```python
from build123d import *

# Parameters (mm, degrees)
F1_DEPTH  = 12.7
F2_R      = 5.08
F3_SIZE   = 6.34999
F7_DEPTH  = 25.4
F9_DEPTH  = 25.4
F6_R      = 3.175
F10_DEPTH = 25.4


# Not quite as in the source:
# - a fillet or chamfer is up to 0.001 mm smaller than in the source, because OpenCascade refuses the exact size


with BuildPart() as f1:
    # F0 (on Top) → F1 (new body)
    with BuildSketch(Plane.XY):
        with BuildLine():
            ThreePointArc((-85.1017062912, 39.9863691127), (36.5051433715, 149.8230416662), (158.1119930343, 39.9863691127))
            Line((158.1119930343, 39.9863691127), (175.5953490648, 40.6241259528))
            ThreePointArc((175.5953490648, 40.6241259528), (36.5051433715, 167.2855416662), (-102.5850623217, 40.6241259528))
            Line((-102.5850623217, 40.6241259528), (-85.1017062912, 39.9863691127))
        make_face()
    extrude(amount=F1_DEPTH)

    # F2
    f2_edges = [f1.edges().sort_by_distance(p)[0] for p in [
        (36.505143, 167.285542, 12.7),
        (36.505143, 167.285542, 0),
    ]]
    fillet(f2_edges, radius=F2_R)

    # F3 (size 6.35 in the source; OpenCascade refuses exactly that, so slightly less here)
    f3_edges = [f1.edges().sort_by_distance(p)[0] for p in [
        (36.505143, 149.823042, 12.7),
        (36.505143, 149.823042, 0),
    ]]
    chamfer(f3_edges, length=F3_SIZE)


with BuildPart() as f4_1:
    # F4: instance of F1
    add(f1.part.mirror(Plane.XY))


with BuildPart() as f1_1:
    add(f1.part)

    # F6 (on face) → F7 (cut)
    with BuildSketch(Plane.XY.offset(12.7)):
        with BuildLine():
            ThreePointArc((163.0583931619, 73.4856437086), (162.4024850501, 75.2552779595), (161.7218329639, 77.0155431585))
            ThreePointArc((161.7218329639, 77.0155431585), (161.8086296648, 75.0304207129), (163.0583931619, 73.4856437086))
        make_face()
    extrude(amount=-F7_DEPTH, mode=Mode.SUBTRACT)

    # F8 (on face) → F9 (cut)
    with BuildSketch(Plane.XY.offset(12.7)):
        with BuildLine():
            ThreePointArc((64.4226124591, 159.2789709622), (62.573664155, 159.6574032574), (60.7195923208, 160.0098780326))
            ThreePointArc((60.7195923208, 160.0098780326), (62.4506994343, 159.0344227782), (64.4226124591, 159.2789709622))
        make_face()
        with BuildLine():
            ThreePointArc((64.4226124591, 159.2789709622), (65.7478153328, 160.450521759), (66.2405230377, 162.1493251742))
            ThreePointArc((66.2405230377, 162.1493251742), (61.9182883246, 165.1098112007), (60.7195923208, 160.0098780326))
            ThreePointArc((60.7195923208, 160.0098780326), (62.573664155, 159.6574032574), (64.4226124591, 159.2789709622))
        make_face()
    extrude(amount=-F9_DEPTH, mode=Mode.SUBTRACT)

    # F6 (on face) → F10 (cut)
    with BuildSketch(Plane.XY.offset(12.7)):
        with Locations((164.7779065912, 76.1547069462)):
            Circle(F6_R)
    extrude(amount=-F10_DEPTH, mode=Mode.SUBTRACT)


solid = f1_1.part
```
Input: part model. Units: mm. Frame: model coordinates. Give positions to 0.01 mm unless a question says otherwise; leave off trailing zeros.
1. Material intervals for L1, parallel to Y at x = 164.5, z = 5.5; L2, parallel to X at y = 47, z = 8.5; L3, parallel to X at y = 99.5, z = 1.5, sorted ascending.
Derived:
L1: y = 40.22 to 72.99, 79.32 to 83.56
L2: x = -101.76 to -86.36, 159.37 to 174.77
L3: x = -81.54 to -68.28, 141.29 to 154.55
2. Mould query, pull axis X, two halves, no side actions, for faces 1 (the conical face through (33.979, 150.105, 6.658)), 2 (the flat face through (-95.91, 40.38, 6.26)), 3 (the flat face through (56, 156, 12.7)), 4 (the flat face through (168.67, 40.37, 6.26)). Classes: released by +X, released by -X, zero draft, split by the parting line, or undercut.
Derived:
face 1: undercut
face 2: released by -X
face 3: zero draft
face 4: released by +X
3. Pin query (flat end, axial travel): pin 1 (6 mm diameter, centred on y = 112, z = 4, fed in from +X); pin 2 (3 mm diameter, centred on x = 64.5, z = 2, fed in from +Y); pin 3 (3 mm diameter, centred on x = 142.5, z = 8.5, fed in from +Y). Return the tip coordinate at first contact, or that it passes through.
Derived:
pin 1: stops at x = 149.96
pin 2: stops at y = 160.94
pin 3: stops at y = 120.22
